Could you check a few things on this model? Use its own coordinates, in mm. A direction names the side the tool comes from. Coordinates: 2 decimals unless noted, no trailing zeros. Order: outer loops, then holes, each group sorted by start corner. A loop starts at its lowest first (then second) coordinate and runs counter-clockwise, first axis right, second up. Notation, with made-up numbers: (62.25, -6.75) - (77.25, -6.75) arc R34 ccw to (77.25, 26.25) - close; hole circle Ø1 at (-10, 2). An arc over 180 degrees is marked (long way). Answer as a JSON object with one key per item and string values. Group by question number.
(1) Imagine slicing it at B-B, the plane z = -1.5. Write out the boundary of the cut face in (x, y).
(2) Please list where these lines run through material, in increasing order: probe 1 along Z at (x, y) = (0, 24) (3 decimals); probe 2 along Z at (x, y) = (6, 0) (3 decimals).
(3) We'd pull the mould along X, two halves only. Please class faces 1 (the cylindrical face through (-12.6, -9.66, 23.02)), 2 (the cylindrical face through (-6.827, 23.017, -10.709)), 3 (the flat face through (-7, 11, 38.1)): pulls with the +X half, pulls with the -X half, needs draft (parallel to the pull), parting line crosses it, or undercut.
(4) Imagine slicing it at C-C, the plane y = 13.5. Write out the boundary of the cut face in (x, z) (3 decimals), and give its area (3 significant figures).
(5) Imagine slicing it at D-D, the plane z = 25.5. Write out the boundary of the cut face in (x, y) (3 decimals), and give its area (3 significant figures).
(6) Which directions (+Z, -Z, +X, -X, +Y, -Y) give clear straight access to the entire face, cutting with the end or side of a thin tool? Please do faces 4 (the flat face through (38.1, 11, 7)), 5 (the cylindrical face through (23.017, -6.08, -14.664)), 6 (the cylindrical face through (-11.7, 23.02, -10.73)).
(7) Imagine slicing it at A-A, the plane y = -8.5. Write out the boundary of the cut face in (x, z), and give its area (3 significant figures).
(8) Will these pins go through, and if not, where does the flat tip stop? P1, Ø8, axis at x = 29, z = 12, coming from the -Y side; P2, Ø1.5, axis at x = 30.5, y = 14, coming from the +Z side; P3, Ø1.5, axis at x = -4.5, z = -4.5, coming from the -Y side.
from build123d import *

# Parameters (mm, degrees)
SKETCH1_R           = 15.875
SKETCH1_R_2         = 12.7
BOSS_EXTRUDE1_DEPTH = 38.1
BOSS_EXTRUDE2_DEPTH = 38.1
SKETCH3_R           = 15.875
SKETCH3_R_2         = 12.7
BOSS_EXTRUDE3_DEPTH = 38.1
REVOLVE1_ANGLE      = 90
SKETCH5_R           = 12.7
CUT_EXTRUDE1_DEPTH  = 38.1
SKETCH6_R           = 12.7
CUT_EXTRUDE2_DEPTH  = 38.1
CUT_EXTRUDE3_START  = -38.1
SKETCH7_R           = 12.7
CUT_EXTRUDE3_DEPTH  = 15.875


with BuildPart() as part:
    # Sketch1 → Boss-Extrude1 (new body)
    with BuildSketch(Plane.XY):
        Circle(SKETCH1_R)
        Circle(SKETCH1_R_2, mode=Mode.SUBTRACT)
    extrude(amount=BOSS_EXTRUDE1_DEPTH)

    # Sketch2 → Boss-Extrude2 (add)
    with BuildSketch(Plane(origin=(0, 0, 0), x_dir=(1, 0, 0), z_dir=(0, 1, 0))):
        with BuildLine():
            ThreePointArc((-15.875, 0), (0, -15.875), (15.875, 0))
            Line((15.875, 0), (12.7, 0))
            ThreePointArc((12.7, 0), (0, -12.7), (-12.7, 0))
            Line((-12.7, 0), (-15.875, 0))
        make_face()
        with BuildLine():
            Line((12.7, 0), (15.875, 0))
            ThreePointArc((15.875, 0), (0, 15.875), (-15.875, 0))
            Line((-15.875, 0), (-12.7, 0))
            ThreePointArc((-12.7, 0), (0, 12.7), (12.7, 0))
        make_face()
        with BuildLine():
            ThreePointArc((-15.875, 0), (0, -15.875), (15.875, 0))
            Line((15.875, 0), (12.7, 0))
            ThreePointArc((12.7, 0), (0, -12.7), (-12.7, 0))
            Line((-12.7, 0), (-15.875, 0))
        make_face()
        with BuildLine():
            Line((12.7, 0), (15.875, 0))
            ThreePointArc((15.875, 0), (0, 15.875), (-15.875, 0))
            Line((-15.875, 0), (-12.7, 0))
            ThreePointArc((-12.7, 0), (0, 12.7), (12.7, 0))
        make_face()
    extrude(amount=BOSS_EXTRUDE2_DEPTH)

    # Sketch3 → Boss-Extrude3 (add)
    with BuildSketch(Plane(origin=(0, 0, 0), x_dir=(0, 0, -1), z_dir=(1, 0, 0))):
        Circle(SKETCH3_R)
        Circle(SKETCH3_R_2, mode=Mode.SUBTRACT)
    extrude(amount=BOSS_EXTRUDE3_DEPTH)

    # Sketch4 → Revolve1 (revolve)
    with BuildSketch(Plane.ZY):
        with BuildLine():
            ThreePointArc((-15.875, 0), (-11.225320151, -11.225320151), (0, -15.875))
            Line((0, -15.875), (0, -12.7))
            ThreePointArc((0, -12.7), (-8.980256121, -8.980256121), (-12.7, 0))
            Line((-12.7, 0), (-15.875, 0))
        make_face()
    revolve(axis=Axis((0, 0, -12.7), (0, 0, -1)), revolution_arc=REVOLVE1_ANGLE)

    # Sketch5 → Cut-Extrude1 (cut)
    with BuildSketch(Plane(origin=(0, 38.1, 0), x_dir=(1, 0, 0), z_dir=(0, 1, 0))):
        Circle(SKETCH5_R)
    extrude(amount=-CUT_EXTRUDE1_DEPTH, mode=Mode.SUBTRACT)

    # Sketch6 → Cut-Extrude2 (cut)
    with BuildSketch(Plane.XY.offset(38.1)):
        Circle(SKETCH6_R)
    extrude(amount=-CUT_EXTRUDE2_DEPTH, mode=Mode.SUBTRACT)

    # Sketch7 → Cut-Extrude3 (cut)
    with BuildSketch(Plane(origin=(38.1, 0, 0), x_dir=(0, 0, -1), z_dir=(1, 0, 0)).offset(CUT_EXTRUDE3_START)):
        Circle(SKETCH7_R)
    extrude(amount=CUT_EXTRUDE3_DEPTH, mode=Mode.SUBTRACT)


solid = part.part
Result set:
{
 "1": {"outline": "(-15.8, 0) arc R15.8 ccw to (0, -15.8) - (38.1, -15.8) - (38.1, -12.61) - (0, -12.61) arc R12.61 cw to (-12.61, 0) - (-12.61, 38.1) - (-15.8, 38.1) - close; (12.61, 12.61) - (38.1, 12.61) - (38.1, 15.8) - (15.8, 15.8) - (15.8, 38.1) - (12.61, 38.1) - close"},
 "2": {"probe 1": "z = -15.875 to -12.7, 12.7 to 15.875", "probe 2": "z = -15.875 to -12.7"},
 "3": {"face 1": "parting line crosses it", "face 2": "undercut", "face 3": "needs draft"},
 "4": {"outline": "(-8.353, 13.5) arc R15.875 ccw (long way) to (13.5, -8.353) - (38.1, -8.353) - (38.1, 8.353) - (13.5, 8.353) arc R15.875 ccw to (8.353, 13.5) - (8.353, 38.1) - (-8.353, 38.1) - close; hole circle Ø25.4 at (0, 0)", "area": "1,050 mm^2"},
 "5": {"outline": "circle Ø31.75 at (0, 0); hole circle Ø25.4 at (0, 0)", "area": "285 mm^2"},
 "6": {"face 4": "+Z, -Z, +X, +Y, -Y", "face 5": "+X", "face 6": "+Y"},
 "7": {"outline": "(-13.41, 0) arc R13.41 ccw to (0, -13.41) - (38.1, -13.41) - (38.1, -9.44) - (0, -9.44) arc R9.44 cw to (-9.44, 0) - (-9.44, 38.1) - (-13.41, 38.1) - close; (9.44, 9.44) - (38.1, 9.44) - (38.1, 13.41) - (13.41, 13.41) - (13.41, 38.1) - (9.44, 38.1) - close", "area": "586 mm^2"},
 "8": {"P1": "stops at y = -13.71", "P2": "stops at z = 8.74", "P3": "stops at y = -14.85"}
}
